CAD build for the part. Positions are in the model's coordinates, mm. Face numbers are marked on the shaded views. A direction names the side the tool comes from. Give positions to 0.01 mm unless a question says otherwise; leave off trailing zeros. Loops run counter-clockwise (first coordinate to the right, second up) from the corner with the lowest first, then second, coordinate; pieces in that order, holes last.
Item 1: Saw through at A-A on x = -40. Give the cut face in (y, z).
Item 2: Probe probe 1 along X at (y, z) = (-2.5, 25.5); probe 2 along X at (y, z) = (-13.75, 31.5); probe 3 along Y at (x, z) = (-43, 37). List the from-to ranges inside material, lowest first.
Item 3: Saw through at B-B on y = -15.25. Give the cut face in (x, z).
Item 4: Saw through at D-D on x = -34.5. Give the cut face in (y, z), plus the area to 3 significant figures.
Item 5: Saw through at C-C on z = 37. Give the cut face in (x, y), plus the area to 3 significant figures.
Item 6: Which spindle directions (+Z, -Z, +X, -X, +Y, -Y) get a long thin tool onto all of the face, cutting with end or side? Do the marked faces 1, 2 and 3. Say none if no direction does.
Item 7: Mould opens along Z. For the marked faces 4, 5 and 6 say: released by +Z, released by -Z, zero draft, split by the parting line, or undercut.
Item 8: Drop flat-ended pins along their axis: P1, Ø1, axis at x = -27.5, y = -11.5, coming from the +Z side; P2, Ø2.5, axis at x = -33, z = 9.5, coming from the +Y side; P3, Ø4, axis at x = -30.5, z = 32.5, coming from the +Y side. Give the stop position or say it passes through.
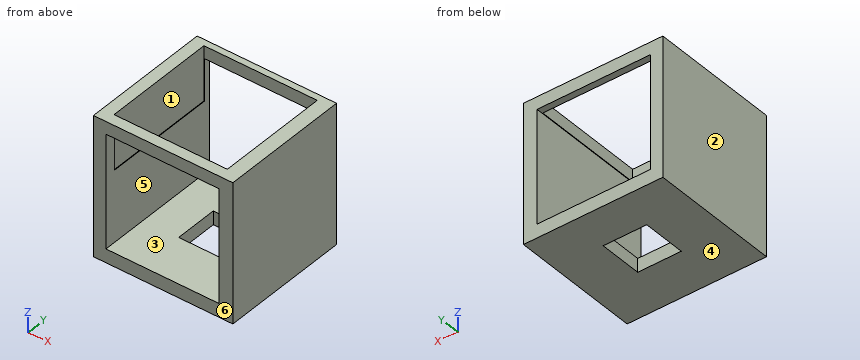
from build123d import *

# Parameters (mm, degrees)
F0_W     = 32
F0_H     = 32
F1_DEPTH = 30
F2_W     = 26
F2_H     = 26
F3_DEPTH = 30.001
F4_W     = 26
F4_H     = 26
F5_DEPTH = 12.5
F6_W     = 10
F6_H     = 10
F7_DEPTH = 32.001


# Not quite as in the source:
# - a feature names something its author has since deleted; it is built from what else it names


with BuildPart() as f1:
    # F0 (on Front) → F1 (new body)
    with BuildSketch(Plane.XZ):
        with Locations((-32.1818544654, 23.1859142184)):
            Rectangle(F0_W, F0_H)
    extrude(amount=F1_DEPTH)

    # F2 (on Front) → F3 (cut, through all)
    with BuildSketch(Plane.XZ):
        with Locations((-32.3113440342, 23.315487102)):
            Rectangle(F2_W, F2_H)
    extrude(amount=F3_DEPTH, mode=Mode.SUBTRACT)

    # F4 (on face) → F5 (cut, symmetric)
    with BuildSketch(Plane.XY.offset(39.1859142184)):
        with Locations((-32.4389154911, -14.4897329509)):
            Rectangle(F4_W, F4_H)
    extrude(amount=F5_DEPTH, both=True, mode=Mode.SUBTRACT)

    # F6 (on face) → F7 (cut, through all)
    with BuildSketch(Plane(origin=(0, 0, 7.1859142184), x_dir=(1, 0, 0), z_dir=(0, 0, -1))):
        with Locations((-32.1818544654, 14.1996787861)):
            Rectangle(F6_W, F6_H)
    extrude(amount=-F7_DEPTH, mode=Mode.SUBTRACT)


solid = f1.part
Results below:
1. outline: (-30, 7.19) - (0, 7.19) - (0, 10.32) - (-30, 10.32) - close; (-30, 36.32) - (-27.49, 36.32) - (-27.49, 39.19) - (-30, 39.19) - close; (-1.49, 36.32) - (0, 36.32) - (0, 39.19) - (-1.49, 39.19) - close
2. probe 1: x = -48.18 to -45.31, -19.31 to -16.18
2. probe 2: x = -48.18 to -45.44, -19.31 to -16.18
2. probe 3: y = -30 to -27.49, -1.49 to 0
3. outline: (-48.18, 7.19) - (-37.18, 7.19) - (-37.18, 10.32) - (-45.31, 10.32) - (-45.31, 26.69) - (-45.44, 26.69) - (-45.44, 39.19) - (-48.18, 39.19) - close; (-27.18, 7.19) - (-16.18, 7.19) - (-16.18, 39.19) - (-19.44, 39.19) - (-19.44, 36.32) - (-19.31, 36.32) - (-19.31, 10.32) - (-27.18, 10.32) - close
4. outline: (-30, 7.19) - (-19.2, 7.19) - (-19.2, 10.32) - (-30, 10.32) - close; (-30, 36.32) - (-27.49, 36.32) - (-27.49, 39.19) - (-30, 39.19) - close; (-9.2, 7.19) - (0, 7.19) - (0, 10.32) - (-9.2, 10.32) - close; (-1.49, 36.32) - (0, 36.32) - (0, 39.19) - (-1.49, 39.19) - close
4. area: 74.1 mm2
5. outline: (-48.18, -30) - (-16.18, -30) - (-16.18, 0) - (-48.18, 0) - close; hole (-45.44, -27.49) - (-19.44, -27.49) - (-19.44, -1.49) - (-45.44, -1.49) - close
5. area: 284 mm2
6. face 1: +Z
6. face 2: +Z, -Z, -X, +Y, -Y
6. face 3: +Y, -Y
7. face 4: released by -Z
7. face 5: undercut
7. face 6: zero draft
8. P1: stops at z = 10.32
8. P2: stops at y = 0
8. P3: passes through
